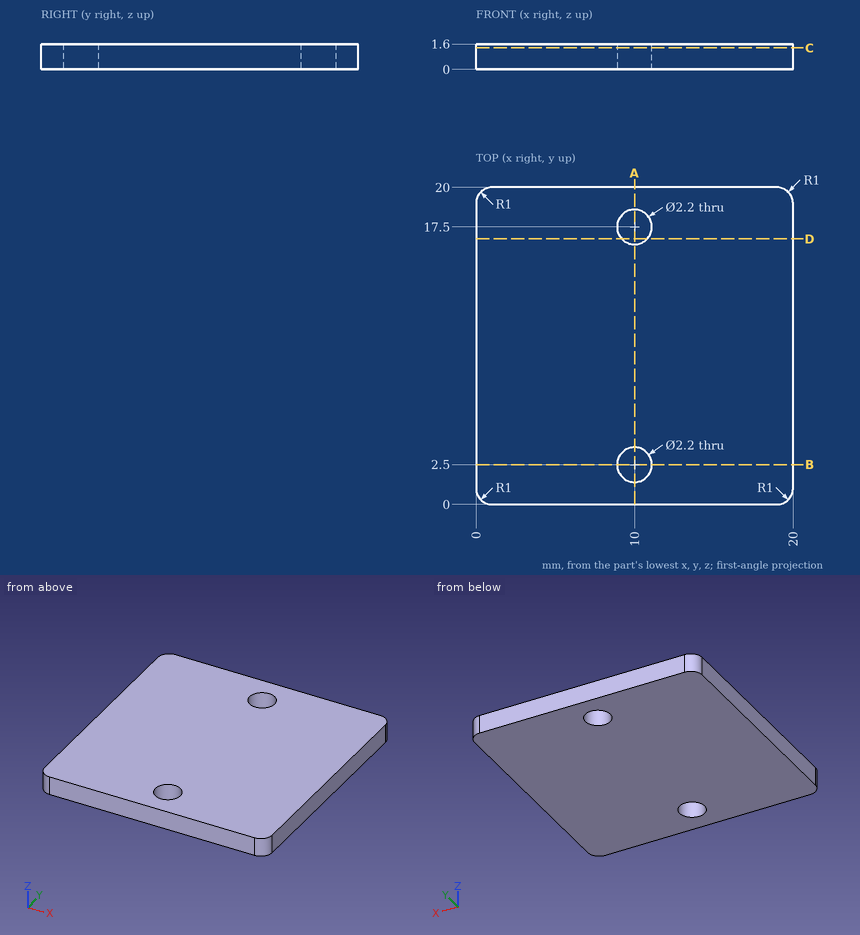
Print and shaded views of the part. All mm, measured from the part's lowest x, y and z. Round coordinates to 2 decimals unless told otherwise and drop trailing zeros. Loops run counter-clockwise (first coordinate to the right, second up) from the corner with the lowest first, then second, coordinate; pieces in that order, holes last. Notation, with made-up numbers: M -23,-22 L 33,-22 A14 ccw 33,5 Z; hole C 79.25,27.25 d5. An arc over 180 degrees is marked long. One line per question, with ' | ' between items.
1) Flat gauge pin, fed straight in: pin 1 (1.8 mm diameter, centred on x = 10, y = 17.5, fed in from -Z) (1 decimal). Where does the tip first touch, or does it go through?
Solved:
pin 1: passes through
2) Band-saw the part on B-B (y = 2.5). Give the cut face in (x, z).
Solved:
outline: M 0,0 L 8.9,0 L 8.9,1.6 L 0,1.6 Z; M 11.1,0 L 20,0 L 20,1.6 L 11.1,1.6 Z
3) Band-saw the part on A-A (x = 10). Give the cut face in (y, z).
Solved:
outline: M 0,0 L 1.4,0 L 1.4,1.6 L 0,1.6 Z; M 3.6,0 L 16.4,0 L 16.4,1.6 L 3.6,1.6 Z; M 18.6,0 L 20,0 L 20,1.6 L 18.6,1.6 Z
4) Drill centre line: line 1 along Y through (x, z) = (10, 1.25). Where is it in solid material? Low to high.
Solved:
line 1: y = 0 to 1.4, 3.6 to 16.4, 18.6 to 20
5) Band-saw the part on D-D (y = 16.75). Give the cut face in (x, z), then the cut area to 3 significant figures.
Solved:
outline: M 0,0 L 9.2,0 L 9.2,1.6 L 0,1.6 Z; M 10.8,0 L 20,0 L 20,1.6 L 10.8,1.6 Z | area: 29.4 mm²
6) Band-saw the part on C-C (z = 1.35). Give the cut face in (x, y).
Solved:
outline: M 0,1 A1 ccw 1,0 L 19,0 A1 ccw 20,1 L 20,19 A1 ccw 19,20 L 1,20 A1 ccw 0,19 Z; hole C 10,2.5 d2.2; hole C 10,17.5 d2.2
